Geometry check sheet. Reference: the model listing, model coordinates, mm. Face numbers are marked on the shaded views. A direction names the side the tool comes from. Coordinates: 2 decimals unless noted, no trailing zeros. Order: outer loops, then holes, each group sorted by start corner. A loop starts at its lowest first (then second) coordinate and runs counter-clockwise, first axis right, second up.
```python
from build123d import *

# Parameters (mm, degrees)
EXTRUDE_THIN1_DEPTH = 25.4
SKETCH3_R           = 2.4765
CUT_EXTRUDE1_DEPTH  = 26.4
SKETCH4_R           = 2.4765
CUT_EXTRUDE2_DEPTH  = 26.4


with BuildPart() as part:
    # Sketch1 → Extrude-Thin1 (new body)
    with BuildSketch(Plane.XY):
        Polygon((25.4, 0), (0, 0), (0, 25.4), (2.54, 25.4), (2.54, 2.54), (25.4, 2.54), align=None)
    extrude(amount=EXTRUDE_THIN1_DEPTH)

    # Sketch3 → Cut-Extrude1 (cut, through all)
    with BuildSketch(Plane.ZY):
        with Locations((12.7, 12.7)):
            Circle(SKETCH3_R)
    extrude(amount=-CUT_EXTRUDE1_DEPTH, mode=Mode.SUBTRACT)

    # Sketch4 → Cut-Extrude2 (cut, through all)
    with BuildSketch(Plane.XZ):
        with Locations((12.7, 12.7)):
            Circle(SKETCH4_R)
    extrude(amount=-CUT_EXTRUDE2_DEPTH, mode=Mode.SUBTRACT)


solid = part.part
```
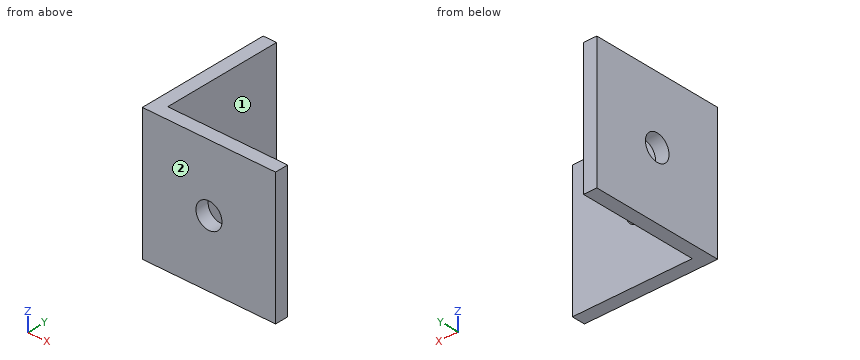
Item 1: Depth check by flat-ended pin: P1, Ø11.5, axis at y = 10, z = 17, coming from the +X side; P2, Ø10, axis at x = 4, y = 21, coming from the +Z side. Enter the tip coordinate at first touch or a pass-through.
Item 2: Sectioned sample at D-D (y = 1.5). Record the cut outline in (x, z), and give its area (3 significant figures).
Item 3: Thickness scan on line 1 along Y through (x, z) = (1.3, 12.7); line 2 along Y through (x, z) = (9.75, 6.25). Record the ranges inside material, lowest first.
Item 4: Tool access check on the marked faces 1 and 2. Record the directions out of +Z, -Z, +X, -X, +Y, -Y that give a thin tool (end or side, any length) a straight path to the whole face; none if there is none.
Item 5: Sectioned sample at A-A (y = 12.7). Record the cut outline in (x, z), and give its area (3 significant figures).
Item 6: Sectioned sample at C-C (z = 12.7). Record the cut outline in (x, y), and give its area (3 significant figures).
Geometry check:
1. P1: stops at x = 2.54
1. P2: stops at z = 25.4
2. outline: (0, 0) - (25.4, 0) - (25.4, 25.4) - (0, 25.4) - close; hole circle Ø4.95 at (12.7, 12.7)
2. area: 626 mm2
3. line 1: y = 0 to 10.22, 15.18 to 25.4
3. line 2: y = 0 to 2.54
4. face 1: +Z, -Z, +X, +Y
4. face 2: +Z, -Z, +X, -X, -Y
5. outline: (0, 0) - (2.54, 0) - (2.54, 10.22) - (0, 10.22) - close; (0, 15.18) - (2.54, 15.18) - (2.54, 25.4) - (0, 25.4) - close
5. area: 51.9 mm2
6. outline: (0, 0) - (10.22, 0) - (10.22, 2.54) - (2.54, 2.54) - (2.54, 10.22) - (0, 10.22) - close; (0, 15.18) - (2.54, 15.18) - (2.54, 25.4) - (0, 25.4) - close; (15.18, 0) - (25.4, 0) - (25.4, 2.54) - (15.18, 2.54) - close
6. area: 97.4 mm2
